from build123d import *

# Parameters (mm, degrees)
SKETCH1_R           = 1.15
SKETCH1_W           = 27.305
SKETCH1_H           = 26.492
SKETCH1_W_2         = 27.241
SKETCH1_H_2         = 3.747
BOSS_EXTRUDE1_DEPTH = 1.5
SKETCH2_W           = 27.241
SKETCH2_H           = 3.747
BOSS_EXTRUDE2_DEPTH = 2
SKETCH3_W           = 27.241
SKETCH3_H           = 3.747
BOSS_EXTRUDE3_DEPTH = 1.5
SKETCH5_W           = 17.241
SKETCH5_H           = 3.747
BOSS_EXTRUDE4_DEPTH = 3
SKETCH6_W           = 27.241
SKETCH6_H           = 3.747
CUT_EXTRUDE1_DEPTH  = 2


with BuildPart() as part:
    # Sketch1 → Boss-Extrude1 (new body)
    with BuildSketch(Plane(origin=(0, 0, 0), x_dir=(1, 0, 0), z_dir=(0, 1, 0))):
        with BuildLine():
            Line((-25.193654123, -23.311779602), (-25.193654123, 28.483220398))
            Line((-25.193654123, 28.483220398), (18.545345877, 28.483220398))
            Line((18.545345877, 28.483220398), (18.545345877, -23.311779602))
            Line((18.545345877, -23.311779602), (18.545345877, -24.511779602))
            Line((18.545345877, -24.511779602), (18.545345877, -25.811779602))
            ThreePointArc((18.545345877, -25.811779602), (17.900980796, -27.367414521), (16.345345877, -28.011779602))
            Line((16.345345877, -28.011779602), (-22.993654123, -28.011779602))
            ThreePointArc((-22.993654123, -28.011779602), (-24.549289041, -27.367414521), (-25.193654123, -25.811779602))
            Line((-25.193654123, -25.811779602), (-25.193654123, -24.511779602))
            Line((-25.193654123, -24.511779602), (-25.193654123, -23.311779602))
        make_face()
        with Locations(Location((-20.164926555, 24.983220398, 0), (0, 0, 270))):
            Circle(SKETCH1_R, mode=Mode.SUBTRACT)
        with Locations(Location((-3.324926555, 24.983220398, 0), (0, 0, 270))):
            Circle(SKETCH1_R, mode=Mode.SUBTRACT)
        with Locations(Location((13.515073445, 24.983220398, 0), (0, 0, 270))):
            Circle(SKETCH1_R, mode=Mode.SUBTRACT)
        with Locations((-3.285420702, -3.096858745)):
            Rectangle(SKETCH1_W, SKETCH1_H, mode=Mode.SUBTRACT)
        with Locations((-0.666632566, 16.558921478)):
            Rectangle(SKETCH1_W_2, SKETCH1_H_2, mode=Mode.SUBTRACT)
    extrude(amount=BOSS_EXTRUDE1_DEPTH)



with BuildPart() as body_2:
    # Sketch2 → Boss-Extrude2 (new body)
    with BuildSketch(Plane(origin=(0, 1.5, 0), x_dir=(1, 0, 0), z_dir=(0, 1, 0))):
        with Locations((-0.666632566, 16.558921478)):
            Rectangle(SKETCH2_W, SKETCH2_H)
    extrude(amount=BOSS_EXTRUDE2_DEPTH)


with BuildPart() as part_1:
    add(part.part)

    add(body_2.part)  # Boss-Extrude3 merges body 2
    # Sketch3 → Boss-Extrude3 (add)
    with BuildSketch(Plane.XZ.offset(-1.5)):
        with Locations((-0.666632566, -16.558921478)):
            Rectangle(SKETCH3_W, SKETCH3_H)
    extrude(amount=BOSS_EXTRUDE3_DEPTH)

    # Sketch5 → Boss-Extrude4 (add)
    with BuildSketch(Plane.XZ):
        with Locations((-0.666632566, -16.558921478)):
            Rectangle(SKETCH5_W, SKETCH5_H)
    extrude(amount=BOSS_EXTRUDE4_DEPTH)

    # Sketch6 → Cut-Extrude1 (cut)
    with BuildSketch(Plane(origin=(0, 3.5, 0), x_dir=(1, 0, 0), z_dir=(0, 1, 0))):
        with Locations((-0.666632566, 16.558921478)):
            Rectangle(SKETCH6_W, SKETCH6_H)
    extrude(amount=-CUT_EXTRUDE1_DEPTH, mode=Mode.SUBTRACT)


solid = part_1.part
Geometry check sheet. Reference: the model listing, model coordinates, mm. A direction names the side the tool comes from. Give positions to 0.01 mm unless a question says otherwise; leave off trailing zeros. Order: outer loops, then holes, each group sorted by start corner. A loop starts at its lowest first (then second) coordinate and runs counter-clockwise, first axis right, second up.
1) Cross-section at A-A (z = 13.5). Record the boundary of the cut face in (x, y).
Results are:
outline: (-25.19, 0) - (-16.94, 0) - (-16.94, 1.5) - (-25.19, 1.5) - close; (10.37, 0) - (18.55, 0) - (18.55, 1.5) - (10.37, 1.5) - close
2) Tool access check on faces 1 (the flat face through (-16.938, 1, 3)), 2 (the flat face through (-1, -1, -18.432)), 3 (the flat face through (-9.287, -1, -17)), 4 (the flat face through (-1, -1, -14.685)). Record the directions out of +Z, -Z, +X, -X, +Y, -Y that give a thin tool (end or side, any length) a straight path to the whole face; none if there is none.
Results are:
face 1: +Y, -Y
face 2: -Z, +X, -X, -Y
face 3: +Z, -Z, -X, -Y
face 4: +Z, +X, -X, -Y
3) Draft check along Z on faces 5 (the flat face through (-3, 1, 16.343)), 6 (the flat face through (-1, -3, -17)), 7 (the cylindrical face through (17.92, 0.74, 27.35)), 8 (the flat face through (-3, 1, -10.149)). Enter one of: released by +Z, released by -Z, zero draft, split by the parting line, or undercut.
Results are:
face 5: undercut
face 6: zero draft
face 7: released by +Z
face 8: undercut
4) Cross-section at C-C (z = -24.5). Record the boundary of the cut face in (x, y), then the cut area to 3 significant figures.
Results are:
outline: (-25.19, 0) - (-21.21, 0) - (-21.21, 1.5) - (-25.19, 1.5) - close; (-19.12, 0) - (-4.37, 0) - (-4.37, 1.5) - (-19.12, 1.5) - close; (-2.28, 0) - (12.47, 0) - (12.47, 1.5) - (-2.28, 1.5) - close; (14.56, 0) - (18.55, 0) - (18.55, 1.5) - (14.56, 1.5) - close
area: 56.2 mm2
5) Material ranges on probe 1 along X at (y, z) = (0.6, 2); probe 2 along X at (y, z) = (1.05, -24.5); probe 3 along Z at (x, y) = (6.5, -2.8), recorded low to high.
Results are:
probe 1: x = -25.19 to -16.94, 10.37 to 18.55
probe 2: x = -25.19 to -21.21, -19.12 to -4.37, -2.28 to 12.47, 14.56 to 18.55
probe 3: z = -18.43 to -14.69
6) Gauge pin test, flat ends, axial feed: pin 1 (2.5 mm diameter, centred on x = -3.32, z = -24.98, fed in from +Y); pin 2 (0.9 mm diameter, centred on y = -2, z = -16, fed in from -X); pin 3 (8 mm diameter, centred on x = -6.5, z = 19, fed in from -Y). Record the tip position at first contact, or that the pin passes through.
Results are:
pin 1: stops at y = 1.5
pin 2: stops at x = -9.29
pin 3: stops at y = 0
7) Cross-section at D-D (z = -16.5). Record the boundary of the cut face in (x, y), then the cut area to 3 significant figures.
Results are:
outline: (-25.19, 0) - (-9.29, 0) - (-9.29, -3) - (7.95, -3) - (7.95, 0) - (18.55, 0) - (18.55, 1.5) - (-25.19, 1.5) - close
area: 117 mm2
8) Cross-section at B-B (x = 9). Record the boundary of the cut face in (y, z), then the cut area to 3 significant figures.
Results are:
outline: (0, -28.48) - (1.5, -28.48) - (1.5, -10.15) - (0, -10.15) - close; (0, 16.34) - (1.5, 16.34) - (1.5, 28.01) - (0, 28.01) - close
area: 45.0 mm2
